from build123d import *

# Parameters (mm, degrees)
F0_R     = 6
F1_DEPTH = 32
F2_W     = 12
F2_H     = 25
F2_H_2   = 15
F3_DEPTH = 30.001


with BuildPart() as f1:
    # F0 (on Front) → F1 (new body)
    with BuildSketch(Plane.XZ):
        with BuildLine():
            Line((15, -86), (15, 0))
            ThreePointArc((15, 0), (-10.323708, 10.882144), (-0.789474, -14.97921))
            ThreePointArc((-0.789474, -14.97921), (1.901905, -16.220677), (3, -18.973666))
            Line((3, -18.973666), (3, -86))
            Line((3, -86), (15, -86))
        make_face()
        Circle(F0_R, mode=Mode.SUBTRACT)
    extrude(amount=F1_DEPTH)

    # F2 (on face) → F3 (cut, through all)
    with BuildSketch(Plane.YZ.offset(15)):
        with BuildLine():
            Line((-22, -45), (-22, -70))
            ThreePointArc((-22, -70), (-16, -76), (-10, -70))
            Line((-10, -70), (-10, -45))
            ThreePointArc((-10, -45), (-16, -39), (-22, -45))
        make_face()
        with Locations((-16, -12.5)):
            Rectangle(F2_W, F2_H)
        with BuildLine():
            ThreePointArc((-16, -86), (-27.313708, -81.313708), (-32, -70))
            Line((-32, -70), (-32, -86))
            Line((-32, -86), (-16, -86))
        make_face()
        with BuildLine():
            Line((0, -86), (0, -70))
            ThreePointArc((0, -70), (-4.686292, -81.313708), (-16, -86))
            Line((-16, -86), (0, -86))
        make_face()
        with Locations((-16, 7.5)):
            Rectangle(F2_W, F2_H_2)
    extrude(amount=-F3_DEPTH, mode=Mode.SUBTRACT)


solid = f1.part
For this review, take the finished solid that the model builds, in its own axes (mm). A direction names the side the tool comes from. Give positions to 0.01 mm unless a question says otherwise; leave off trailing zeros. Write each loop counter-clockwise with the first axis right and the second up, starting at its lowest first coordinate (ties: lowest second). Pieces come first, ordered by that corner, then holes. Notation, with made-up numbers: (80.5, 41) -> (110.5, 41) arc R16 cw to (110.5, 59) -> close; hole circle Ø8 at (79, 41). An arc over 180 degrees is marked (long way). Use CSV: the item, a comma, the result in double quotes.
Q1. Mouldability with a two-part tool opening along Z and no side actions: class faces 6 (the face through (3, -32, -17)), 7 (the face through (1.87, -26.93, -16.19)), 8 (the face through (9, -22, -57)) as pulls with the +Z half, pulls with the -Z half, needs draft (parallel to the pull), parting line crosses it, or undercut.
Conclusion:
face 6,"needs draft"
face 7,"pulls with the -Z half"
face 8,"undercut"
Q2. To check wall thickness, follow probe 1 along Y at (x, z) = (-11.5, -6.5); probe 2 along X at (y, z) = (-27, 0); probe 3 along Z at (x, y) = (0, -27.25). State the ranges of each line that lie inside material, in increasing order. Write a range as [from, to].
Conclusion:
probe 1,"[-32, -22], [-10, 0]"
probe 2,"[-15, -6], [6, 15]"
probe 3,"[-15.1, -6], [6, 15]"
Q3. Take a section at A-A, the plane z = -54.5. Write out the cut boundary in (x, y).
Conclusion:
outline,"(3, -32) -> (15, -32) -> (15, -22) -> (3, -22) -> close; (3, -10) -> (15, -10) -> (15, 0) -> (3, 0) -> close"
Q4. Tool access review of faces 1 (the face through (-6, -27, 0)), 2 (the face through (3, -23, -52)), 3 (the face through (9, -16, -76)), 4 (the face through (3, 0, -17)), 5 (the face through (4, -10, -5)): name each direction out of +Z, -Z, +X, -X, +Y, -Y from which nothing blocks a thin tool from reaching the whole face with its end or side.
Conclusion:
face 1,"+Y, -Y"
face 2,"-Z, -X, +Y, -Y"
face 3,"+X, -X"
face 4,"+Z, -Z, +X, -X, +Y"
face 5,"+Z, +X, -X"
Q5. Take a section at B-B, the plane x = 1. Write out the cut boundary in (y, z), then the cut area to 3 significant figures.
Conclusion:
outline,"(-32, -15.51) -> (-22, -15.51) -> (-22, -5.92) -> (-32, -5.92) -> close; (-32, 5.92) -> (-22, 5.92) -> (-22, 14.97) -> (-32, 14.97) -> close; (-10, -15.51) -> (0, -15.51) -> (0, -5.92) -> (-10, -5.92) -> close; (-10, 5.92) -> (0, 5.92) -> (0, 14.97) -> (-10, 14.97) -> close"
area,"373 mm2"
Q6. For P1, Ø1.5, axis at x = -8, y = -4.5, coming from the +Z side; P2, Ø8, axis at x = 6.5, y = -23, coming from the -Z side; P3, Ø9.5, axis at y = -10.5, z = -39, coming from the -X side, all flat-tipped, find the tip position at first contact; note any pin that passes through.
Conclusion:
P1,"z = 13.13"
P2,"z = -85.72"
P3,"x = 3"
Q7. Take a section at C-C, the plane y = -18. Write out the cut boundary in (x, z), then the cut area to 3 significant figures.
Conclusion:
outline,"(3, -85.87) -> (15, -85.87) -> (15, -75.66) -> (3, -75.66) -> close; (3, -39.34) -> (15, -39.34) -> (15, -25) -> (3, -25) -> close"
area,"295 mm2"
Q8. Take a section at D-D, the plane y = -4. Write out the cut boundary in (x, z).
Conclusion:
outline,"(-0.79, -14.98) arc R4 cw to (3, -18.97) -> (3, -80.58) -> (15, -80.58) -> (15, 0) arc R15 ccw (long way) to start; hole circle Ø12 at (0, 0)"
